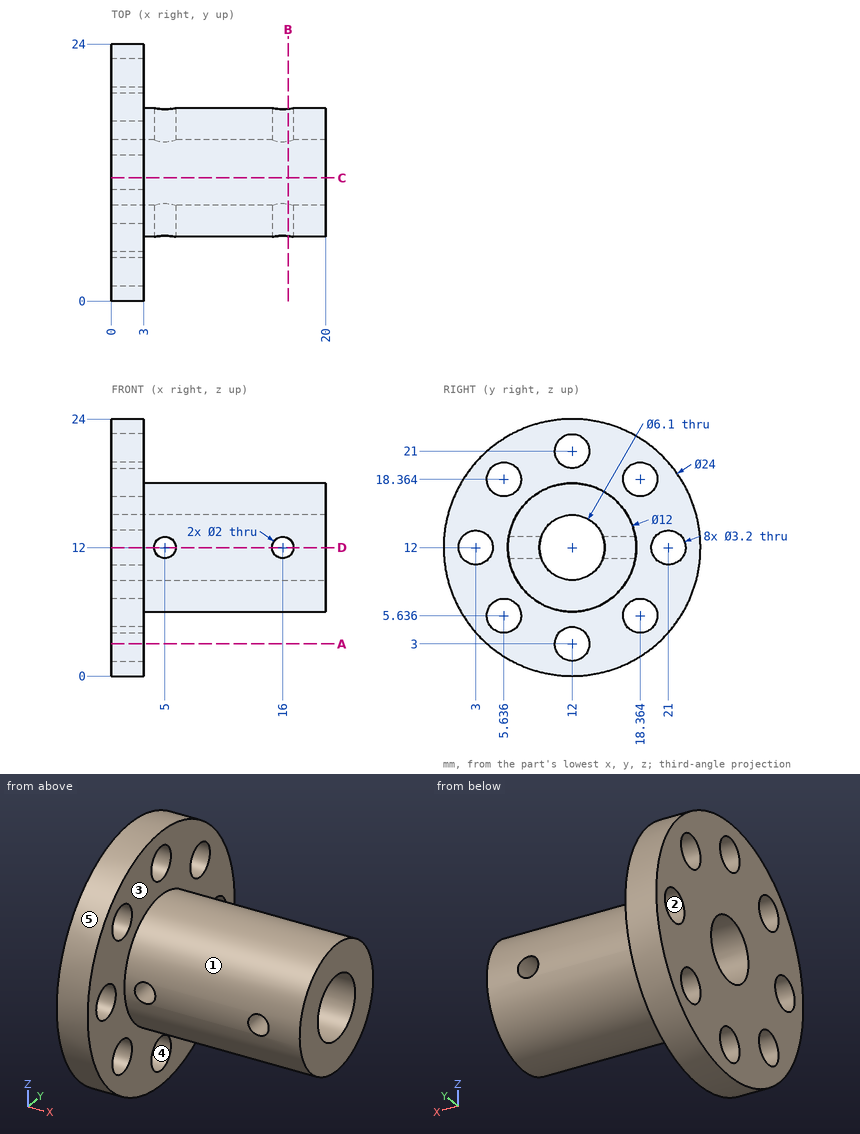
Here's the drawing with two shaded views (mm, measured from the low corner). I have some questions. A direction names the side the tool comes from. Give positions to 0.01 mm unless a question says otherwise; leave off trailing zeros. Order: outer loops, then holes, each group sorted by start corner. A loop starts at its lowest first (then second) coordinate and runs counter-clockwise, first axis right, second up. Notation, with made-up numbers: (60, 47) - (88, 47) arc R19 ccw to (88, 61) - close; hole circle Ø7 at (-10, 32.25). An arc over 180 degrees is marked (long way). Use a Markdown table: item, result. Add a question column.
Q1. On a 3-axis mill with a long thin cutter (end or side, diameter ignored), from which of +Z, -Z, +X, -X, +Y, -Y can I reach the whole of each face in a straight line? I mean the marked faces 1 and 2. Say none if no direction works.
Q2. If we section it at B-B on x = 16.5: Write out the boundary of the cut face in (y, z).
Q3. If we section it at D-D on z = 12: Count the separate pieces of the cut face and the enclosed holes in it, plus the area to 3 significant figures.
Q4. Please list where these lines run through material, in increasing order: line 1 along X through (y, z) = (17.4, 12); line 2 along Y through (x, z) = (1, 11); line 3 along Z through (x, y) = (2.25, 18).
Q5. If we mould it in two halves opening along Z, with no side actions, what happens to the marked faces 3, 4 and 5? For each: released by +Z, released by -Z, zero draft, split by the parting line, or undercut.
Q6. If we section it at C-C on y = 11.5: Write out the boundary of the cut face in (x, z).
Q7. If we section it at A-A on z = 3: Write out the boundary of the cut face in (x, y).
Q8. I'm going to push flat-ended pins straight in: pin 1 (3.5 mm diameter, centred on y = 12, z = 12, fed in from -X); pin 2 (5 mm diameter, centred on y = 3, z = 12, fed in from -X); pin 3 (2.5 mm diameter, centred on x = 5, z = 12, fed in from +Y); pin 4 (5 mm diameter, centred on x = 8, y = 12.5, fed in from +Z). Where does each tip first touch, or does it pass through?
Answers follow:
| question | item | result |
|---|---|---|
| 1 | face 1 | +X |
| 1 | face 2 | +X, -X |
| 2 | outline | (6.06, 11.13) arc R6 ccw to (17.94, 11.13) - (14.92, 11.13) arc R3.05 cw to (9.08, 11.13) - close; (6.06, 12.87) - (9.08, 12.87) arc R3.05 cw to (14.92, 12.87) - (17.94, 12.87) arc R6 ccw to start |
| 3 | separate pieces | 8 |
| 3 | enclosed holes | 0 |
| 3 | area | 111 mm^2 |
| 4 | line 1 | x = 0 to 4, 6 to 15, 17 to 20 |
| 4 | line 2 | y = 0.04 to 1.75, 4.25 to 9.12, 14.88 to 19.75, 22.25 to 23.96 |
| 4 | line 3 | z = 1.61 to 4.08, 7.19 to 16.81, 19.92 to 22.39 |
| 5 | face 3 | zero draft |
| 5 | face 4 | undercut |
| 5 | face 5 | split by the parting line |
| 6 | outline | (0, 0.01) - (3, 0.01) - (3, 1.48) - (0, 1.48) - close; (0, 4.52) - (3, 4.52) - (3, 6.02) - (20, 6.02) - (20, 8.99) - (0, 8.99) - close; (0, 15.01) - (20, 15.01) - (20, 17.98) - (3, 17.98) - (3, 19.48) - (0, 19.48) - close; (0, 22.52) - (3, 22.52) - (3, 23.99) - (0, 23.99) - close |
| 7 | outline | (0, 4.06) - (3, 4.06) - (3, 10.4) - (0, 10.4) - close; (0, 13.6) - (3, 13.6) - (3, 19.94) - (0, 19.94) - close |
| 8 | pin 1 | passes through |
| 8 | pin 2 | stops at x = 0 |
| 8 | pin 3 | stops at y = 18 |
| 8 | pin 4 | stops at z = 18 |
